Geometry: final body of the model. Coordinates: model frame, mm. A direction names the side the tool comes from. Give positions to 0.01 mm unless a question says otherwise; leave off trailing zeros. Write each loop counter-clockwise with the first axis right and the second up, starting at its lowest first coordinate (ties: lowest second). Pieces come first, ordered by that corner, then holes. Notation, with made-up numbers: M 2,75.5 L 28,75.5 A14 ccw 28,83.5 Z; hole C -1.5,36.25 d10. An arc over 180 degrees is marked long. Answer as a JSON object with one key per item and string values.
from build123d import *

# Parameters (mm, degrees)
SKETCH_1_W          = 16
SKETCH_1_H          = 6
EXTRUDE_1_DEPTH     = 2
SKETCH_1_3_W        = 16
SKETCH_1_3_H        = 2
SKETCH_1_3_H_2      = 1.5
EXTRUDE_2_DEPTH     = 15
SKETCH_2_W          = 8
SKETCH_2_H          = 26
CUT_EXTRUDE_1_DEPTH = 2
EXTRUDE_3_DEPTH     = 2.5
EXTRUDE_4_DEPTH     = 5
EXTRUDE_5_DEPTH     = 1.5
SKETCH_9_W          = 1.2
SKETCH_9_H          = 1.820432063
EXTRUDE_6_DEPTH     = 2
EXTRUDE_7_DEPTH     = 12
CUT_EXTRUDE_START   = -7.10494
CUT_EXTRUDE_2_DEPTH = 7.10494
SKETCH_12_R         = 1.281793471
CUT_EXTRUDE_3_DEPTH = 10
CUT_EXTRUDE_4_DEPTH = 20.2
SKETCH_14_W         = 5.2
SKETCH_14_H         = 1
EXTRUDE_8_DEPTH     = 30
SKETCH_14_2_W       = 5.2
SKETCH_14_2_H       = 1
EXTRUDE_9_DEPTH     = 12
SKETCH_15_W         = 1
SKETCH_15_H         = 16
EXTRUDE_10_DEPTH    = 16
CHAMFER_1_SIZE      = 3


with BuildPart() as part:
    # 草图1 → 凸台-拉伸1 (new body)
    with BuildSketch(Plane(origin=(0, 0, 0), x_dir=(1, 0, 0), z_dir=(0, 1, 0))):
        with Locations((0, -0.25)):
            Rectangle(SKETCH_1_W, SKETCH_1_H)
    extrude(amount=EXTRUDE_1_DEPTH)

    # 草图1<3> → 凸台-拉伸2 (add)
    with BuildSketch(Plane(origin=(0, 0, 0), x_dir=(1, 0, 0), z_dir=(0, 1, 0))):
        with Locations((0, 3.75)):
            Rectangle(SKETCH_1_3_W, SKETCH_1_3_H)
        with Locations((0, -4)):
            Rectangle(SKETCH_1_3_W, SKETCH_1_3_H_2)
    extrude(amount=EXTRUDE_2_DEPTH)

    # 草图2 → 切除-拉伸1 (cut)
    with BuildSketch(Plane(origin=(0, 0, -4.75), x_dir=(-1, 0, 0), z_dir=(0, 0, -1))):
        with Locations((0, 15)):
            Rectangle(SKETCH_2_W, SKETCH_2_H)
    extrude(amount=-CUT_EXTRUDE_1_DEPTH, mode=Mode.SUBTRACT)

    # 草图3 → 凸台-拉伸3 (add, symmetric)
    with BuildSketch(Plane(origin=(0, 0, 0), x_dir=(0, 0, -1), z_dir=(1, 0, 0))):
        Polygon((4.75, 0), (8.831597644, 0), (11.768525918, 13.935665169), (4.75, 15.414812878), align=None)
    extrude(amount=EXTRUDE_3_DEPTH, both=True)

    # 草图5 → 凸台-拉伸4 (add)
    with BuildSketch(Plane(origin=(2.5, 0, 0), x_dir=(0, 0, -1), z_dir=(1, 0, 0))):
        Polygon((4.75, 6.451105389), (3.822798244, 8.744995241), (3.822798244, 15.463750373), (4.75, 15.414812878), align=None)
    extrude(amount=-EXTRUDE_4_DEPTH)

    # 草图6 → 凸台-拉伸5 (add)
    with BuildSketch(Plane.ZY.offset(2.5)):
        Polygon((-4.75, 6.451105389), (-10.094945569, 5.994560313), (-11.768525918, 13.935665169), (-4.75, 15.414812878), (-3.822798244, 15.463750373), (-3.822798244, 8.744995241), align=None)
    extrude_5 = extrude(amount=EXTRUDE_5_DEPTH)

    # 草图9 → 凸台-拉伸6 (add)
    with BuildSketch(Plane.XZ):
        with Locations((8.6, -2.660216032)):
            Rectangle(SKETCH_9_W, SKETCH_9_H)
        with Locations((-8.6, -2.660216032)):
            Rectangle(SKETCH_9_W, SKETCH_9_H)
    extrude(amount=-EXTRUDE_6_DEPTH)

    # 草图9<3> → 凸台-拉伸7 (add)
    with BuildSketch(Plane.XZ):
        Polygon((8, -3.570432063), (8, -4.75), (11.2, -4.75), (11.2, -1.75), (9.2, -1.75), (9.2, -3.570432063), align=None)
        Polygon((-8, -4.75), (-8, -3.570432063), (-9.2, -3.570432063), (-9.2, -1.75), (-11.2, -1.75), (-11.2, -4.75), align=None)
    extrude(amount=-EXTRUDE_7_DEPTH)

    # 草图11 → 切除-拉伸2 (cut)
    with BuildSketch(Plane(origin=(0, -1.782098659, -8.456022034), x_dir=(-1, 0, 0), z_dir=(0, -0.206219179, -0.978505825)).offset(CUT_EXTRUDE_START)):
        Polygon((2.5, 7.947483572), (4, 11.245323919), (4, 7.947483572), (4, 5.815044055), (2.5, 5.815044055), align=None)
    cut_extrude_2 = extrude(amount=CUT_EXTRUDE_2_DEPTH, mode=Mode.SUBTRACT)

    # 镜向1: 凸台-拉伸5, 切除-拉伸2 across plane
    add(extrude_5.mirror(Plane(origin=(0, 0, 0), x_dir=(0, 0, 1), z_dir=(1, 0, 0))))
    add(cut_extrude_2.mirror(Plane(origin=(0, 0, 0), x_dir=(0, 0, 1), z_dir=(1, 0, 0))), mode=Mode.SUBTRACT)

    # 草图12 → 切除-拉伸3 (cut)
    with BuildSketch(Plane(origin=(4, 0, 0), x_dir=(0, 0, -1), z_dir=(1, 0, 0))):
        with Locations((9.183579002, 11.7521089)):
            Circle(SKETCH_12_R)
    extrude(amount=-CUT_EXTRUDE_3_DEPTH, mode=Mode.SUBTRACT)

    # 草图13 → 切除-拉伸4 (cut, through all)
    with BuildSketch(Plane(origin=(8, 0, 0), x_dir=(0, 0, -1), z_dir=(1, 0, 0))):
        Polygon((-3.25, 9.484512334), (-4.55, 9.484512334), (-4.55, 0), (-4.75, 0), (-4.75, 15), (-3.25, 15), align=None)
    extrude(amount=-CUT_EXTRUDE_4_DEPTH, mode=Mode.SUBTRACT)

    # 草图14 → 凸台-拉伸8 (add)
    with BuildSketch(Plane(origin=(0, 12, 0), x_dir=(1, 0, 0), z_dir=(0, 1, 0))):
        with Locations((10.6, 4.25)):
            Rectangle(SKETCH_14_W, SKETCH_14_H)
        with Locations((-10.6, 4.25)):
            Rectangle(SKETCH_14_W, SKETCH_14_H)
    extrude(amount=EXTRUDE_8_DEPTH)

    # 草图14<2> → 凸台-拉伸9 (add)
    with BuildSketch(Plane(origin=(0, 12, 0), x_dir=(1, 0, 0), z_dir=(0, 1, 0))):
        with Locations((10.6, 4.25)):
            Rectangle(SKETCH_14_2_W, SKETCH_14_2_H)
        with Locations((-10.6, 4.25)):
            Rectangle(SKETCH_14_2_W, SKETCH_14_2_H)
    extrude(amount=-EXTRUDE_9_DEPTH)

    # 草图15 → 凸台-拉伸10 (add)
    with BuildSketch(Plane(origin=(-8, 0, 0), x_dir=(0, 0, -1), z_dir=(1, 0, 0))):
        with Locations((4.25, 34)):
            Rectangle(SKETCH_15_W, SKETCH_15_H)
    extrude(amount=EXTRUDE_10_DEPTH)

    # 倒角1
    chamfer_1_edges = [part.edges().sort_by_distance(p)[0] for p in [
        (-8, 26, -4.25),
        (8, 26, -4.25),
    ]]
    chamfer(chamfer_1_edges, length=CHAMFER_1_SIZE)


solid = part.part
1) Cut plane A-A on x = -6.5. Return loops of the section in (y, z).
Geometry check:
{"outline": "M 0,-4.75 L 15,-4.75 L 15,-2.75 L 2,-2.75 L 2,3.25 L 9.48,3.25 L 9.48,4.55 L 0,4.55 Z; M 24.5,-4.75 L 42,-4.75 L 42,-3.75 L 24.5,-3.75 Z"}
2) Cut plane C-C on z = -6.5. Return loops of the section in (x, y), and give its area (3 significant figures).
Geometry check:
{"outline": "M -4,10.12 L -2.5,6.75 L -2.5,0 L 2.5,0 L 2.5,6.75 L 4,10.12 L 4,15.05 L -4,15.05 Z", "area": "95.1 mm2"}
3) Contact query for flat-ended pins moving along their axis: P1, Ø2, axis at x = -8.5, y = 31, coming from the +Z side; P2, Ø1.7, axis at y = 2, z = -7, coming from the +X side; P3, Ø1.1, axis at y = 9.5, z = -3, coming from the +X side; P4, Ø1, axis at x = 1.5, y = 17.5, coming from the -Z side. Output: stop coordinate, or through.
Geometry check:
{"P1": "stops at z = -3.75", "P2": "stops at x = 2.5", "P3": "stops at x = 11.2", "P4": "passes through"}
4) Cut plane B-B on x = 0. Return loops of the section in (y, z) (3 decimals).
Geometry check:
{"outline": "M 0,-8.832 L 13.936,-11.769 L 15.415,-4.75 L 15.464,-3.823 L 8.745,-3.823 L 6.451,-4.75 L 2,-4.75 L 2,3.25 L 9.485,3.25 L 9.485,4.55 L 0,4.55 Z; M 26,-4.75 L 42,-4.75 L 42,-3.75 L 26,-3.75 Z; hole C 11.752,-9.184 d2.564"}
5) Cut plane D-D on x = 10. Return loops of the section in (y, z), and give its area (3 significant figures).
Geometry check:
{"outline": "M 0,-4.75 L 42,-4.75 L 42,-3.75 L 12,-3.75 L 12,-1.75 L 0,-1.75 Z", "area": "66.0 mm2"}
6) Set-up query: faces 1 (the flat face through (4, 7, -4)), 2 (the flat face through (6, 25, -4)), 3 (the flat face through (0, 0, -1)), 4 (the flat face through (0, 9.485, 4)). Return all of +Z, -Z, +X, -X, +Y, -Y with unobstructed straight access to the full face (end or side cutting, diameter ignored); none if empty.
Geometry check:
{"face 1": "none", "face 2": "+Z, -Z", "face 3": "+Z, -Z, +X, -X, -Y", "face 4": "+Z, +X, -X, +Y"}
7) Pull-direction query (X, two-part tool) for faces 5 (the flat face through (10, 6, -1.75)), 6 (the flat face through (11.2, 6, -3)), 7 (the flat face through (-13.2, 21, -4)), 8 (the flat face through (-8, 8, -3)); classes: pulls with the +X half, pulls with the -X half, needs draft (parallel to the pull), parting line crosses it, or undercut.
Geometry check:
{"face 5": "needs draft", "face 6": "pulls with the +X half", "face 7": "pulls with the -X half", "face 8": "undercut"}
8) Line query: line 1 (Y direction, x = -3.25, z = 2.5); line 2 (Z direction, x = -12, y = 31); line 3 (Z direction, x = 8.75, y = 8). Output: solid intervals per line, ascending. Write a range as from..to.
Geometry check:
{"line 1": "y = 0..2", "line 2": "z = -4.75..-3.75", "line 3": "z = -4.75..-3.57"}
